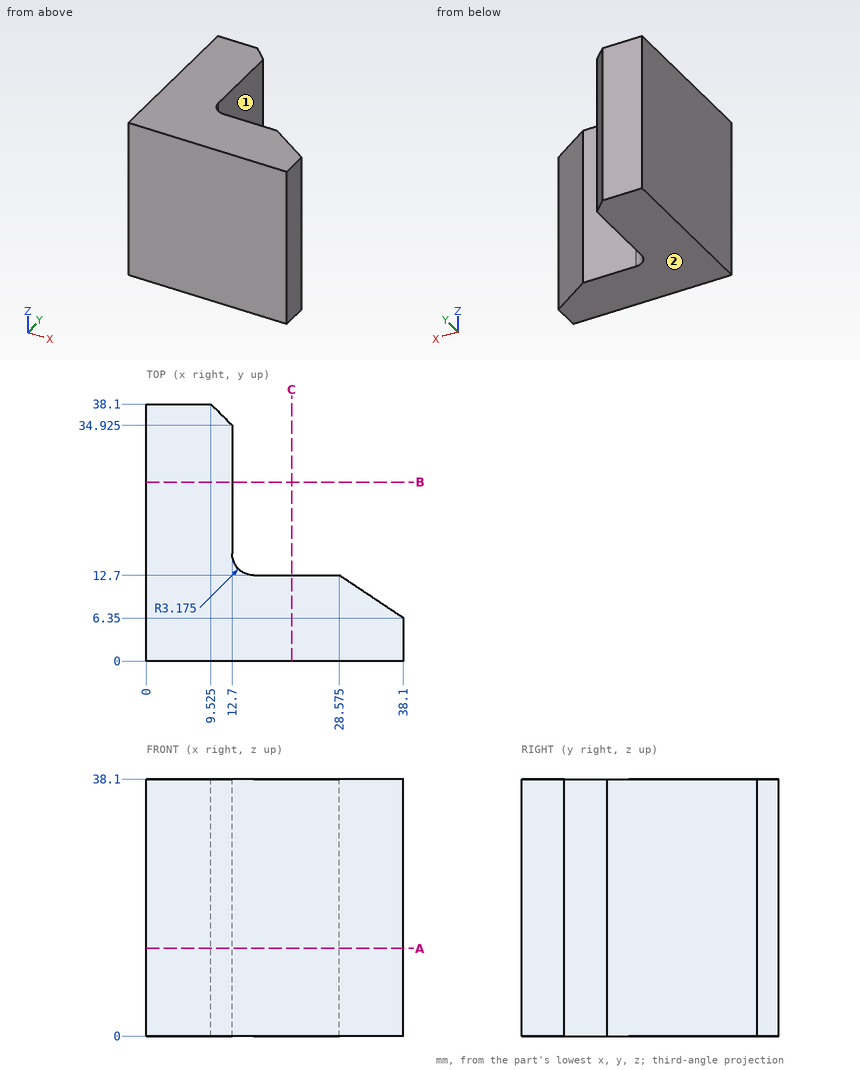
Study the drawing (mm; zero at the part's minimum x, y, z) and answer. A direction names the side the tool comes from. Round coordinates to 2 decimals unless told otherwise and drop trailing zeros. Order: outer loops, then holes, each group sorted by start corner. A loop starts at its lowest first (then second) coordinate and runs counter-clockwise, first axis right, second up. Notation, with made-up numbers: M -5,77.25 L 53,77.25 A12 ccw 53,94.25 Z; hole C 14,-9 d11. An arc over 180 degrees is marked long. One line per item, written item: value.
Q1. For the marked faces 1 and 2, determine the directions among +Z, -Z, +X, -X, +Y, -Y from which every point of the face is accessible in a straight line to the end or side of a thin tool.
Derived:
face 1: +Z, -Z, +X, +Y
face 2: -Z, +X, -X, +Y, -Y
Q2. Flat-ended cylindrical pins translate along their axes: pin 1 (1.5 mm diameter, centred on x = 17, z = 23, fed in from +Y); pin 2 (2 mm diameter, centred on y = 31, z = 26, fed in from +X); pin 3 (3 mm diameter, centred on y = 10, z = 17, fed in from +X) (3 decimals). Find the tip coordinate at first contact, or state that the pin passes through.
Derived:
pin 1: y = 12.7
pin 2: x = 12.7
pin 3: x = 34.875
Q3. Find section B-B on y = 26.5. Write down the section's boundary in (x, z), then the cut area to 3 significant figures.
Derived:
outline: M 0,0 L 12.7,0 L 12.7,38.1 L 0,38.1 Z
area: 484 mm²
Q4. Straight lines are drawn through the part: line 1 (X direction, y = 33, z = 2); line 2 (X direction, y = 11.5, z = 21) (3 decimals). For each, find the intervals that lie inside material, in ascending order.
Derived:
line 1: 0 to 12.7
line 2: 0 to 30.375
Q5. Find section A-A on z = 13. Write down the section's boundary in (x, y) (3 decimals).
Derived:
outline: M 0,0 L 38.1,0 L 38.1,6.35 L 28.575,12.7 L 15.875,12.7 A3.175 cw 12.7,15.875 L 12.7,34.925 L 9.525,38.1 L 0,38.1 Z
